Geometry check sheet. Reference: the model listing, model coordinates, mm. Give positions to 0.01 mm unless a question says otherwise; leave off trailing zeros. Loops run counter-clockwise (first coordinate to the right, second up) from the corner with the lowest first, then second, coordinate; pieces in that order, holes last.
1. Cross-section at A-A, the plane y = 17.75. Record the cut outline in (x, z).
2. Release check for a two-part mould opening along Z. For faces 1 (the cylindrical face through (12.63, 15.876, 2.563)), 2 (the flat face through (13, 9, 0)), 3 (the cylindrical face through (12.522, 4.702, 18.734)) record: +Z half, -Z half, draft (parallel to the pull), parting line (faces both ways), or undercut.
3. Cross-section at B-B, the plane x = 12.7. Record the cut outline in (y, z) (3 decimals).
4. Material ranges on L1, parallel to Z at x = 20.5, y = 10.75; L2, parallel to Z at x = 21.5, y = 6.5; L3, parallel to Y at x = 2.5, z = 26, recorded low to high.
5. Cross-section at C-C, the plane z = 35. Record the cut outline in (x, y) (3 decimals), plus the area to 3 significant figures.
6. Cross-section at D-D, the plane z = 19.05. Record the cut outline in (x, y), plus the area to 3 significant figures.
Autodesk Fusion 360 part; units mm, degrees
sketch "Sketch1" plane through (0, 0, 0) normal (1, 0, 0) x (0, 1, 0)
  line L0 (19.05, 38.1) -> (0, 38.1)
  line L1 (0, 38.1) -> (0, 0)
  line L2 (0, 0) -> (19.05, 0)
  line L3 (19.05, 0) -> (19.05, 4.699)
  line L4 (19.05, 38.1) -> (19.05, 33.401)
  line L5 (19.05, 33.401) -> (19.05, 4.699) construction
  arc A0 (19.05, 33.401) -> (19.05, 4.699) centre (19.05, 19.05) ccw
  dimension "d1" = 14.351
  dimension "d3" = 19.05
  dimension "d4" = 38.1
extrude "Extrude1" add sketch "Sketch1" along normal blind 25.4
sketch "Sketch2" plane through (0, 0, 38.1) normal (0, 0, 1) x (-1, 0, 0)
  line L0 (0, -19.05) -> (0, 0)
  line L1 (0, 0) -> (-25.4, 0)
  line L2 (-25.4, 0) -> (-25.4, -19.05)
  line L3 (-25.4, -19.05) -> (0, -19.05)
  circle A0 centre (-12.7, -19.05) radius 3.175
  dimension "d7" = 6.35
extrude "Extrude2" cut sketch "Sketch2" against normal up to surface (38.1 mm away) contours L3 A0 | L3 A0
Result:
1. outline: (0, 0) - (9.8, 0) - (9.8, 4.76) - (0, 4.76) - close; (0, 33.34) - (9.8, 33.34) - (9.8, 38.1) - (0, 38.1) - close; (15.6, 0) - (25.4, 0) - (25.4, 4.76) - (15.6, 4.76) - close; (15.6, 33.34) - (25.4, 33.34) - (25.4, 38.1) - (15.6, 38.1) - close
2. face 1: draft
2. face 2: -Z half
2. face 3: undercut
3. outline: (0, 0) - (15.875, 0) - (15.875, 5.055) arc R14.351 cw to (15.875, 33.045) - (15.875, 38.1) - (0, 38.1) - close
4. L1: z = 0 to 7.34, 30.76 to 38.1
4. L2: z = 0 to 12.09, 26.01 to 38.1
4. L3: y = 0 to 6.49
5. outline: (0, 0) - (25.4, 0) - (25.4, 19.05) - (15.875, 19.05) arc R3.175 cw to (9.525, 19.05) - (0, 19.05) - close
5. area: 468 mm2
6. outline: (0, 0) - (25.4, 0) - (25.4, 4.7) - (0, 4.7) - close
6. area: 119 mm2
